CAD build for the part. Positions are in the model's coordinates, mm. A direction names the side the tool comes from. Round coordinates to 2 decimals unless told otherwise and drop trailing zeros. Write each loop counter-clockwise with the first axis right and the second up, starting at its lowest first coordinate (ties: lowest second). Pieces come first, ordered by that corner, then holes. Notation, with made-up numbers: (29, -36.5) - (84, -36.5) arc R18 ccw to (84, -7.5) - close; hole circle Ø9 at (20, -14.5). An arc over 180 degrees is marked (long way). Put each result on its own line as item: value. Start each with the question number.
Item 1: Cut at B-B (z = -32.5). Give the cut face in (x, y).
Item 2: Mould opens along Z. For faces 6 (the flat face through (85.25, 11, 68)), 7 (the flat face through (-83, 11, -70.25)), 8 (the flat face through (-83, 11, -65.75)) say: released by +Z, released by -Z, zero draft, split by the parting line, or undercut.
Item 3: Cut at C-C (x = 64.5). Give the cut face in (y, z).
Item 4: Drill centre lines: line 1 (Z direction, x = 83, y = 12.75); line 2 (Z direction, x = -75, y = 1.45); line 3 (X direction, y = 2.05, z = -60). Where is each one in solid material? Low to high. Write a range as from..to.
Item 5: Cut at A-A (y = 11.5). Give the cut face in (x, z).
Item 6: 3-axis set-ups, long thin cutter, end or side, ignore diameter. For faces 1 (the flat face through (-83, 11, 70.25)), 2 (the flat face through (85.25, 11, -68)), 3 (the flat face through (-85.25, 11, -68)), 4 (the flat face through (-84.1, 1.5, 69.5)), 5 (the flat face through (-84, 1.5, -70)): which of +Z, -Z, +X, -X, +Y, -Y reach the whole face in a straight line?
Item 7: Pin check, flat tips, straight feed: pin 1 Ø3.5 at (y, z) = (9.5, 69) entering from -X; pin 2 Ø5 at (x, y) = (-84, 11.5) entering from +Z; pin 3 Ø5 at (x, y) = (82, 9) entering from -Z. Stop position of each tip, or through.
```python
from build123d import *

# Parameters (mm, degrees)
SKETCH1_W           = 172
SKETCH1_H           = 142
SKETCH1_R           = 1.6
BOSS_EXTRUDE1_DEPTH = 3
SKETCH1_3_W         = 4.5
SKETCH1_3_H         = 4.5
SKETCH1_3_R         = 1.6
BOSS_EXTRUDE2_DEPTH = 20
SKETCH1_5_W         = 4.7
SKETCH1_5_H         = 0.65
SKETCH1_5_H_2       = 4.7
SKETCH1_5_W_2       = 4.5
SKETCH1_5_H_3       = 4.5
SKETCH1_5_R         = 1.6
CUT_EXTRUDE1_DEPTH  = 1.5


with BuildPart() as part:
    # Sketch1 → Boss-Extrude1 (new body)
    with BuildSketch(Plane(origin=(0, 0, 0), x_dir=(1, 0, 0), z_dir=(0, 1, 0))):
        Rectangle(SKETCH1_W, SKETCH1_H)
        with Locations(Location((-75, 60, 0), (0, 0, 270))):
            Circle(SKETCH1_R, mode=Mode.SUBTRACT)
        with Locations(Location((75, 60, 0), (0, 0, 270))):
            Circle(SKETCH1_R, mode=Mode.SUBTRACT)
        with Locations(Location((75, -60, 0), (0, 0, 270))):
            Circle(SKETCH1_R, mode=Mode.SUBTRACT)
        with Locations(Location((-75, -60, 0), (0, 0, 270))):
            Circle(SKETCH1_R, mode=Mode.SUBTRACT)
        with Locations(Location((-83, 68, 0), (0, 0, 270))):
            Circle(SKETCH1_R, mode=Mode.SUBTRACT)
        with Locations(Location((83, 68, 0), (0, 0, 270))):
            Circle(SKETCH1_R, mode=Mode.SUBTRACT)
        with Locations(Location((83, -68, 0), (0, 0, 270))):
            Circle(SKETCH1_R, mode=Mode.SUBTRACT)
        with Locations(Location((-83, -68, 0), (0, 0, 90))):
            Circle(SKETCH1_R, mode=Mode.SUBTRACT)
    extrude(amount=BOSS_EXTRUDE1_DEPTH)

    # Sketch1_3 → Boss-Extrude2 (add)
    with BuildSketch(Plane(origin=(0, 0, 0), x_dir=(1, 0, 0), z_dir=(0, 1, 0))):
        with Locations((-83, -68)):
            Rectangle(SKETCH1_3_W, SKETCH1_3_H)
        with Locations(Location((-83, -68, 0), (0, 0, 90))):
            Circle(SKETCH1_3_R, mode=Mode.SUBTRACT)
        with Locations((83, -68)):
            Rectangle(SKETCH1_3_W, SKETCH1_3_H)
        with Locations(Location((83, -68, 0), (0, 0, 270))):
            Circle(SKETCH1_3_R, mode=Mode.SUBTRACT)
        with Locations((83, 68)):
            Rectangle(SKETCH1_3_W, SKETCH1_3_H)
        with Locations(Location((83, 68, 0), (0, 0, 270))):
            Circle(SKETCH1_3_R, mode=Mode.SUBTRACT)
        with Locations((-83, 68)):
            Rectangle(SKETCH1_3_W, SKETCH1_3_H)
        with Locations(Location((-83, 68, 0), (0, 0, 270))):
            Circle(SKETCH1_3_R, mode=Mode.SUBTRACT)
    extrude(amount=BOSS_EXTRUDE2_DEPTH)

    # Sketch1_5 → Cut-Extrude1 (cut)
    with BuildSketch(Plane(origin=(0, 0, 0), x_dir=(1, 0, 0), z_dir=(0, 1, 0))):
        with Locations((83, 70.675)):
            Rectangle(SKETCH1_5_W, SKETCH1_5_H)
        with Locations((83, 68)):
            Rectangle(SKETCH1_5_W, SKETCH1_5_H_2)
        with Locations((83, 68)):
            Rectangle(SKETCH1_5_W_2, SKETCH1_5_H_3, mode=Mode.SUBTRACT)
        with Locations((83, 68)):
            Rectangle(SKETCH1_5_W_2, SKETCH1_5_H_3)
        with Locations(Location((83, 68, 0), (0, 0, 270))):
            Circle(SKETCH1_5_R, mode=Mode.SUBTRACT)
        with Locations((-83, 68)):
            Rectangle(SKETCH1_5_W, SKETCH1_5_H_2)
        with Locations((-83, 68)):
            Rectangle(SKETCH1_5_W_2, SKETCH1_5_H_3, mode=Mode.SUBTRACT)
        with Locations((-83, 68)):
            Rectangle(SKETCH1_5_W_2, SKETCH1_5_H_3)
        with Locations(Location((-83, 68, 0), (0, 0, 270))):
            Circle(SKETCH1_5_R, mode=Mode.SUBTRACT)
        with Locations((-83, 70.675)):
            Rectangle(SKETCH1_5_W, SKETCH1_5_H)
        with Locations((-83, -68)):
            Rectangle(SKETCH1_5_W, SKETCH1_5_H_2)
        with Locations((-83, -68)):
            Rectangle(SKETCH1_5_W_2, SKETCH1_5_H_3, mode=Mode.SUBTRACT)
        with Locations((-83, -68)):
            Rectangle(SKETCH1_5_W_2, SKETCH1_5_H_3)
        with Locations(Location((-83, -68, 0), (0, 0, 270))):
            Circle(SKETCH1_5_R, mode=Mode.SUBTRACT)
        with Locations((-83, -70.675)):
            Rectangle(SKETCH1_5_W, SKETCH1_5_H)
        with Locations((83, -70.675)):
            Rectangle(SKETCH1_5_W, SKETCH1_5_H)
        with Locations((83, -68)):
            Rectangle(SKETCH1_5_W, SKETCH1_5_H_2)
        with Locations((83, -68)):
            Rectangle(SKETCH1_5_W_2, SKETCH1_5_H_3, mode=Mode.SUBTRACT)
        with Locations((83, -68)):
            Rectangle(SKETCH1_5_W_2, SKETCH1_5_H_3)
        with Locations(Location((83, -68, 0), (0, 0, 270))):
            Circle(SKETCH1_5_R, mode=Mode.SUBTRACT)
    extrude(amount=CUT_EXTRUDE1_DEPTH, mode=Mode.SUBTRACT)


solid = part.part
```
Output values:
1. outline: (-86, 0) - (86, 0) - (86, 3) - (-86, 3) - close
2. face 6: zero draft
2. face 7: released by -Z
2. face 8: undercut
3. outline: (0, -71) - (3, -71) - (3, 71) - (0, 71) - close
4. line 1: -70.25..-69.6, -66.4..-65.75, 65.75..66.4, 69.6..70.25
4. line 2: -71..-61.6, -58.4..58.4, 61.6..71
4. line 3: -86..-76.6, -73.4..73.4, 76.6..86
5. outline: (-85.25, -70.25) - (-80.75, -70.25) - (-80.75, -65.75) - (-85.25, -65.75) - close; (-85.25, 65.75) - (-80.75, 65.75) - (-80.75, 70.25) - (-85.25, 70.25) - close; (80.75, -70.25) - (85.25, -70.25) - (85.25, -65.75) - (80.75, -65.75) - close; (80.75, 65.75) - (85.25, 65.75) - (85.25, 70.25) - (80.75, 70.25) - close; hole circle Ø3.2 at (-83, -68); hole circle Ø3.2 at (-83, 68); hole circle Ø3.2 at (83, -68); hole circle Ø3.2 at (83, 68)
6. face 1: +Z, +X, -X, +Y
6. face 2: +Z, -Z, +X, +Y
6. face 3: +Z, -Z, -X, +Y
6. face 4: +Z, -Y
6. face 5: -Z, -Y
7. pin 1: x = -85.25
7. pin 2: z = 70.25
7. pin 3: z = -70.25
